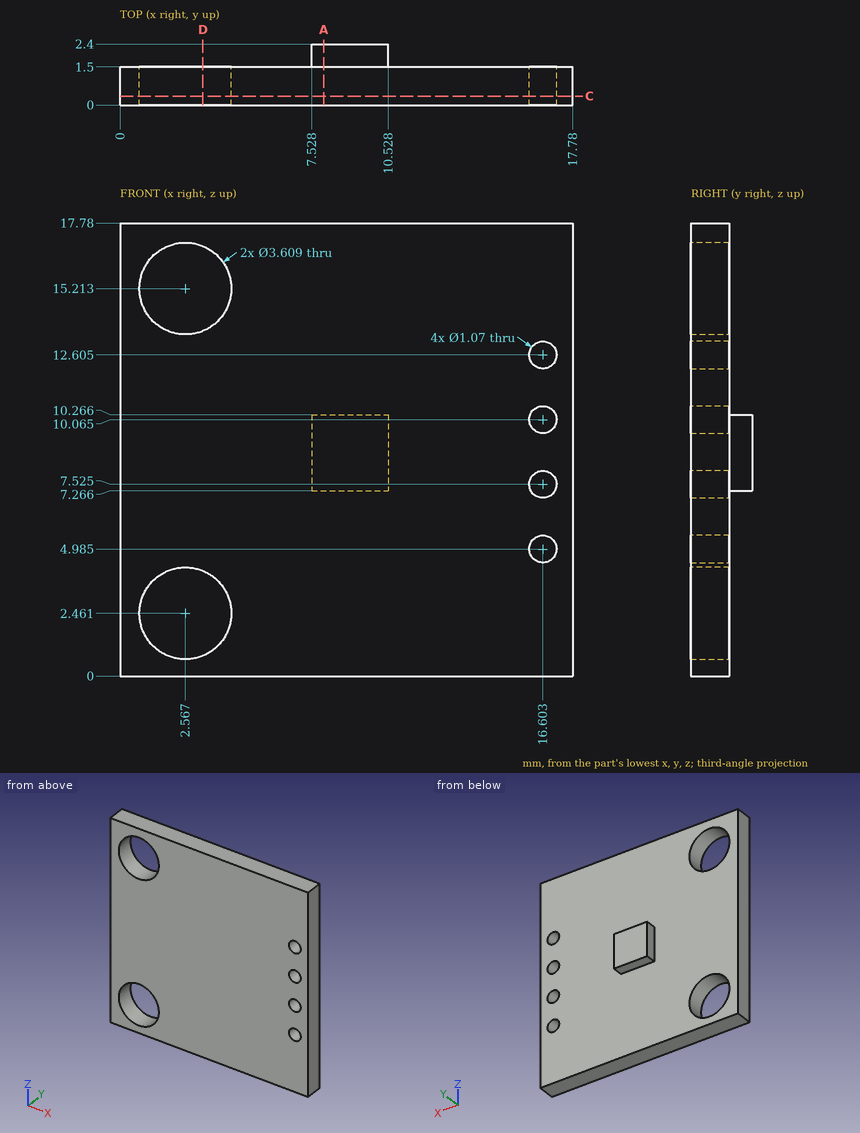
Source: three-view drawing plus pictorial views. Frame: mm from the lowest corner of the part. Give positions to 0.01 mm unless a question says otherwise; leave off trailing zeros. Loops run counter-clockwise (first coordinate to the right, second up) from the corner with the lowest first, then second, coordinate; pieces in that order, holes last.
1) Section query D-D on x = 3.25. Return the cut outline in (y, z).
A:
outline: (0, 0) - (1.5, 0) - (1.5, 0.79) - (0, 0.79) - close; (0, 4.13) - (1.5, 4.13) - (1.5, 13.54) - (0, 13.54) - close; (0, 16.88) - (1.5, 16.88) - (1.5, 17.78) - (0, 17.78) - close
2) Line query: L1, parallel to Z at x = 2.5, y = 1.1 (1 decimal); L2, parallel to X at y = 0.4, z = 5; L3, parallel to X at y = 0.45, z = 2.5. Output: solid intervals per line, ascending.
A:
L1: z = 0 to 0.7, 4.3 to 13.4, 17 to 17.8
L2: x = 0 to 16.07, 17.14 to 17.78
L3: x = 0 to 0.76, 4.37 to 17.78
3) Section query A-A on x = 8. Return the cut outline in (y, z).
A:
outline: (0, 0) - (1.5, 0) - (1.5, 7.27) - (2.4, 7.27) - (2.4, 10.27) - (1.5, 10.27) - (1.5, 17.78) - (0, 17.78) - close
4) Section query C-C on y = 0.35. Return the cut outline in (x, z) (1 decimal).
A:
outline: (0, 0) - (17.8, 0) - (17.8, 17.8) - (0, 17.8) - close; hole circle Ø3.6 at (2.6, 2.5); hole circle Ø3.6 at (2.6, 15.2); hole circle Ø1.1 at (16.6, 5); hole circle Ø1.1 at (16.6, 7.5); hole circle Ø1.1 at (16.6, 10.1); hole circle Ø1.1 at (16.6, 12.6)
5) Contact query for flat-ended pins moving along their axis: pin 1 (0.9 mm diameter, centred on x = 16.6, z = 7.53, fed in from -Y); pin 2 (0.7 mm diameter, centred on y = 2, z = 8.5, fed in from +X); pin 3 (5 mm diameter, centred on x = 2, z = 2.5, fed in from +Y). Output: stop coordinate, or through.
A:
pin 1: passes through
pin 2: stops at x = 10.53
pin 3: stops at y = 1.5
